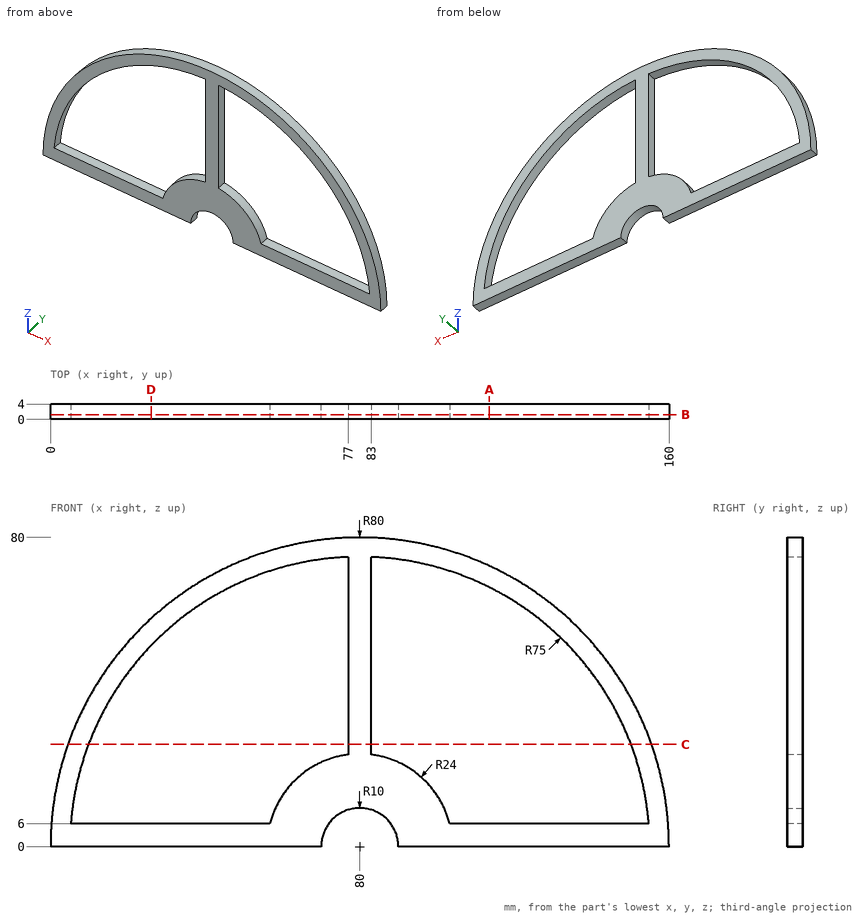
Study the drawing (mm; zero at the part's minimum x, y, z) and answer. Give positions to 0.01 mm unless a question says otherwise; leave off trailing zeros. Order: outer loops, then holes, each group sorted by start corner. A loop starts at its lowest first (then second) coordinate and runs counter-clockwise, first axis right, second up.
1) Find section C-C on z = 26.5. Write down the section's boundary in (x, y), then the cut area to 3 significant figures.
Reported:
outline: (4.52, 0) - (9.84, 0) - (9.84, 4) - (4.52, 4) - close; (77, 0) - (83, 0) - (83, 4) - (77, 4) - close; (150.16, 0) - (155.48, 0) - (155.48, 4) - (150.16, 4) - close
area: 66.6 mm2
2) Find section A-A on x = 113.5. Write down the section's boundary in (y, z).
Reported:
outline: (0, 0) - (4, 0) - (4, 6) - (0, 6) - close; (0, 67.1) - (4, 67.1) - (4, 72.65) - (0, 72.65) - close
3) Given P1, Ø8, axis at x = 16, z = 33, coming from the +Y side; P2, Ø1.2, axis at y = 1.5, z = 38, coming from the -X side; P3, Ø2, axis at x = 137.5, y = 3, coming from the +Z side; P4, Ø1, axis at y = 0.5, z = 67.5, coming from the +X side (3 decimals), each flat-ended and moving along its own axis, determine where each tip first touches the part or whether it passes through.
Reported:
P1: stops at y = 4
P2: stops at x = 9.28
P3: stops at z = 56.64
P4: stops at x = 123.715
4) Consider line 1 along X through (y, z) = (2.1, 65.5); line 2 along X through (y, z) = (2.05, 19); line 3 along Z through (x, y) = (80, 2.55). Determine where each line is inside the solid, lowest interval first.
Reported:
line 1: x = 34.07 to 43.47, 77 to 83, 116.53 to 125.93
line 2: x = 2.29 to 7.45, 65.34 to 94.66, 152.55 to 157.71
line 3: z = 10 to 80
5) Find section D-D on x = 26. Write down the section's boundary in (y, z), then the cut area to 3 significant figures.
Reported:
outline: (0, 0) - (4, 0) - (4, 6) - (0, 6) - close; (0, 52.05) - (4, 52.05) - (4, 59.03) - (0, 59.03) - close
area: 51.9 mm2
6) Find section B-B on y = 1.25. Write down the section's boundary in (x, z).
Reported:
outline: (0, 0) - (70, 0) arc R10 cw to (90, 0) - (160, 0) arc R80 ccw to start; hole (5.24, 6) - (56.76, 6) arc R24 cw to (77, 23.81) - (77, 74.94) arc R75 ccw to start; hole (83, 23.81) arc R24 cw to (103.24, 6) - (154.76, 6) arc R75 ccw to (83, 74.94) - close
